Can you work these out from the drawing? Everything is in mm from the part's minimum corner. A direction names the side the tool comes from. Round coordinates to 2 decimals unless told otherwise and drop trailing zeros. Loops run counter-clockwise (first coordinate to the right, second up) from the corner with the lowest first, then second, coordinate; pieces in that order, holes last. Notation, with made-up numbers: (22, 64) -> (80, 64) arc R25 cw to (80, 91) -> close; hole circle Ø2 at (41.25, 39). An arc over 180 degrees is marked (long way). One line per item, written item: value.
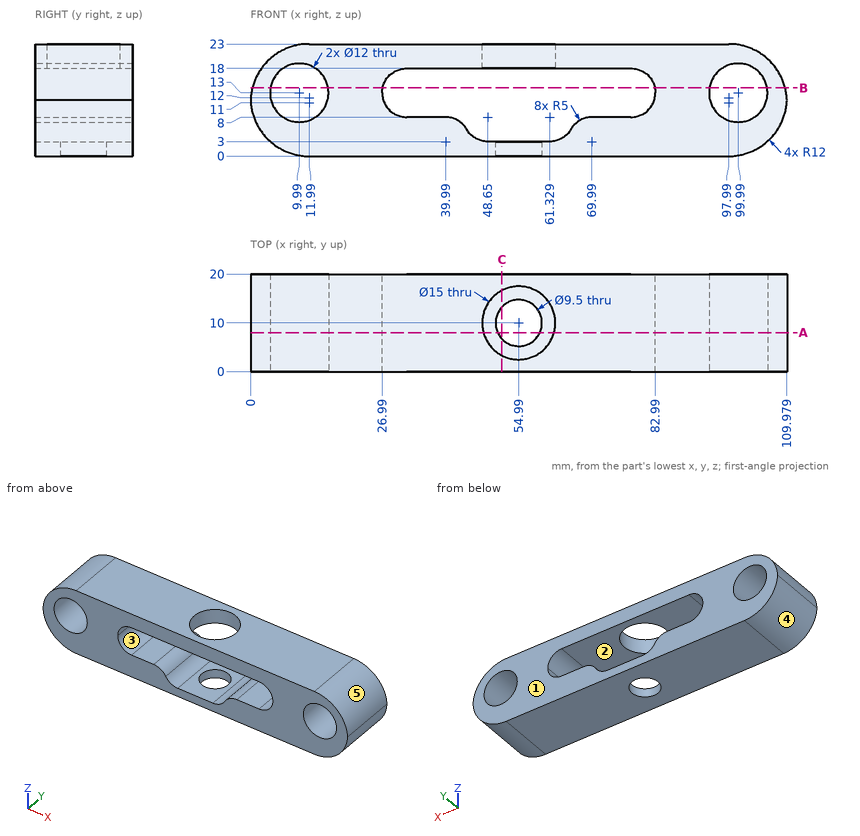
Item 1: If we section it at B-B on z = 14: List the corners of the cut face in (x, y) for me (1 decimal).
Output:
outline: (0.4, 0) -> (4.1, 0) -> (4.1, 20) -> (0.4, 20) -> close; (15.9, 0) -> (27.1, 0) -> (27.1, 20) -> (15.9, 20) -> close; (82.9, 0) -> (94.1, 0) -> (94.1, 20) -> (82.9, 20) -> close; (105.9, 0) -> (109.6, 0) -> (109.6, 20) -> (105.9, 20) -> close
Item 2: If we section it at C-C on x = 51.5: List the corners of the cut face in (y, z) for me.
Output:
outline: (0, 0) -> (6.78, 0) -> (6.78, 3) -> (0, 3) -> close; (0, 18) -> (3.36, 18) -> (3.36, 23) -> (0, 23) -> close; (13.22, 0) -> (20, 0) -> (20, 3) -> (13.22, 3) -> close; (16.64, 18) -> (20, 18) -> (20, 23) -> (16.64, 23) -> close
Item 3: If we section it at A-A on y = 8: Count the separate pieces of the cut face and the enclosed holes in it, plus the area to 3 significant figures.
Output:
separate pieces: 2
enclosed holes: 2
area: 1,440 mm²
Item 4: For the marked faces 1 and 2, which set-ups out of +Z, -Z, +X, -X, +Y, -Y let a thin tool reach every point of the face, with its end or its side?
Output:
face 1: +Z, -Z, +X, -X, +Y
face 2: +Y, -Y
Item 5: I need wall thicknesses on line 1 (X direction, y = 14.75, z = 13.75) (1 decimal); line 2 (X direction, y = 6.25, z = 14.5); line 3 (Z direction, x = 34.5, y = 10.25). Which ranges of each line are inside material? Lowest first, please. Write a range as from..to.
Output:
line 1: x = 0.3..4, 15.9..27, 82.9..94, 105.9..109.7
line 2: x = 0.51..4.18, 15.8..27.22, 82.76..94.18, 105.8..109.47
line 3: z = 0..8, 18..23
Item 6: Will these pins go through, and if not, where does the flat tip stop? pin 1 Ø8.5 at (x, y) = (54.99, 10) entering from -Z; pin 2 Ø1 at (y, z) = (17.5, 2.5) entering from +X (1 decimal); pin 3 Ø6 at (y, z) = (10.5, 5) entering from -X (1 decimal).
Output:
pin 1: passes through
pin 2: stops at x = 105.9
pin 3: stops at x = 0.7
Item 7: If we mould it in two halves opening along Z, with no side actions, what happens to the marked faces 3, 4 and 5? For each: released by +Z, released by -Z, zero draft, split by the parting line, or undercut.
Output:
face 3: undercut
face 4: released by -Z
face 5: released by +Z
